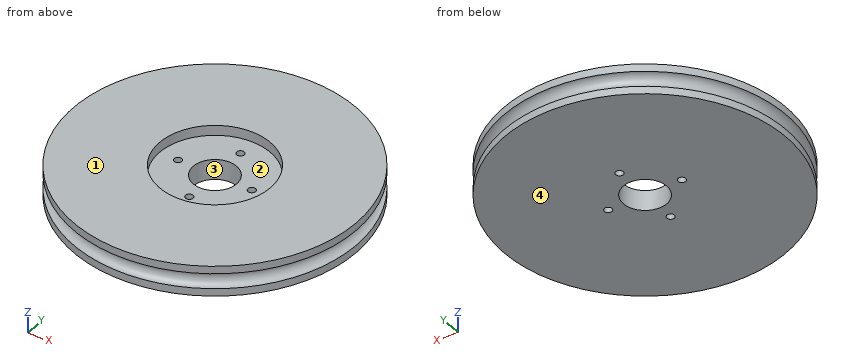
from build123d import *

# Parameters (mm, degrees)
CYLINDER003_R     = 0.75
CYLINDER003_DEPTH = 10
ARRAY_COUNT       = 4
CYLINDER002_R     = 4.3
CYLINDER002_DEPTH = 10
CYLINDER001_R     = 11
CYLINDER001_DEPTH = 10
TORUS_R           = 1.5
CYLINDER_R        = 28
CYLINDER_DEPTH    = 6


with BuildPart() as array:
    # Cylinder003 → Cylinder003 (new body)
    with BuildSketch(Plane(origin=(7.3, 0, -5), x_dir=(1, 0, 0), z_dir=(0, 0, 1))):
        Circle(CYLINDER003_R)
    extrude(amount=CYLINDER003_DEPTH)

    # Array: Array ×4 about axis
    array_axis = Axis((0, 0, 0), (0, 0, 1))


with BuildPart() as array_1:
    add(array.part)
    for i in range(1, ARRAY_COUNT):
        add(array.part.rotate(array_axis, i * 360 / ARRAY_COUNT))


with BuildPart() as hueco_del_eje:
    # Cylinder002 → Cylinder002 (new body)
    with BuildSketch(Plane.XY.offset(-4)):
        Circle(CYLINDER002_R)
    extrude(amount=CYLINDER002_DEPTH)


with BuildPart() as corona_servo:
    # Cylinder001 → Cylinder001 (new body)
    with BuildSketch(Plane.XY.offset(1)):
        Circle(CYLINDER001_R)
    extrude(amount=CYLINDER001_DEPTH)


with BuildPart() as obj1:
    # Torus → Torus (revolve)
    with BuildSketch(Plane.XZ):
        with Locations((28, 0)):
            Circle(TORUS_R)
    revolve(axis=Axis((0, 0, 0), (0, 0, 1)))


with BuildPart() as obj2:
    # Cylinder → Cylinder (new body)
    with BuildSketch(Plane.XY.offset(-3)):
        Circle(CYLINDER_R)
    extrude(amount=CYLINDER_DEPTH)

    # Cut: cut obj1
    add(obj1.part, mode=Mode.SUBTRACT)

    # Cut001: cut Corona servo
    add(corona_servo.part, mode=Mode.SUBTRACT)

    # Cut002: cut Hueco del eje
    add(hueco_del_eje.part, mode=Mode.SUBTRACT)

    # Cut003: cut Array
    add(array_1.part, mode=Mode.SUBTRACT)


solid = obj2.part
Source: CAD feature listing. Evaluate the final solid. Frame: model axes, mm. Face numbers are marked on the shaded views. A direction names the side the tool comes from. Give positions to 0.01 mm unless a question says otherwise; leave off trailing zeros. Write each loop counter-clockwise with the first axis right and the second up, starting at its lowest first coordinate (ties: lowest second). Pieces come first, ordered by that corner, then holes. Notation, with made-up numbers: M 38.25,7.5 L 56.25,7.5 A27 cw 56.25,37.5 Z; hole C -29,62 d7. An arc over 180 degrees is marked long. Return JSON: item names as keys, results as strings. Group by question number.
1) Ray query, L1, parallel to Y at x = 2, z = 0.45; L2, parallel to Y at x = 7.3, z = -1.35; L3, parallel to Z at x = 22, y = 17. Return the intervals inside material, ascending.
2) Cut plane A-A, the plane z = -0.7. Output: boundary loops of the cut face in (x, y), then the cut area to 3 significant figures.
3) First-contact query: pin 1 Ø1.7 at (x, y) = (0, 7.3) entering from +Z; pin 2 Ø1.4 at (x, y) = (0, -7.3) entering from +Z. Flat tips, straight axial feed; report the tip coordinate or a pass-through.
4) Draft query along X for the marked faces 3 and 4. Return one class per face: released by +X, released by -X, zero draft, split by the parting line, or undercut.
5) Set-up query: the marked faces 1 and 2. Return all of +Z, -Z, +X, -X, +Y, -Y with unobstructed straight access to the full face (end or side cutting, diameter ignored); none if empty.
6) Cut plane B-B, the plane z = 2.2. Output: boundary loops of the cut face in (x, y).
Data:
{
 "1": {"L1": "y = -26.49 to -3.81, 3.81 to 26.49", "L2": "y = -26.35 to -0.75, 0.75 to 26.35", "L3": "z = -3 to -1.49, 1.49 to 3"},
 "2": {"outline": "C 0,0 d53.35; hole C -7.3,0 d1.5; hole C 0,0 d8.6; hole C 0,-7.3 d1.5; hole C 0,7.3 d1.5; hole C 7.3,0 d1.5", "area": "2,170 mm²"},
 "3": {"pin 1": "stops at z = 1", "pin 2": "passes through"},
 "4": {"face 3": "undercut", "face 4": "zero draft"},
 "5": {"face 1": "+Z, +X, -X, +Y, -Y", "face 2": "+Z"},
 "6": {"outline": "C 0,0 d56; hole C 0,0 d22"}
}
